```python
from build123d import *

# Parameters (mm, degrees)
EXTRUDE_1_DEPTH = 9.6
DRAFT_5_ANGLE   = -15


with BuildPart() as part:
    # 草图1 → 凸台-拉伸1 (new body)
    with BuildSketch(Plane.XY):
        Polygon((9.8, 0), (0, 0), (0, -108.97), (49.6, -108.97), (49.6, 0), (39.8, 0), (39.8, -10), (9.8, -10), align=None)
    extrude(amount=EXTRUDE_1_DEPTH)

    # 拔模5
    draft_5_faces = [part.faces().sort_by_distance(p)[0] for p in [
        (24.8, -10, 4.8),
    ]]
    draft(draft_5_faces, Plane.XY.offset(9.6), DRAFT_5_ANGLE)


solid = part.part
```
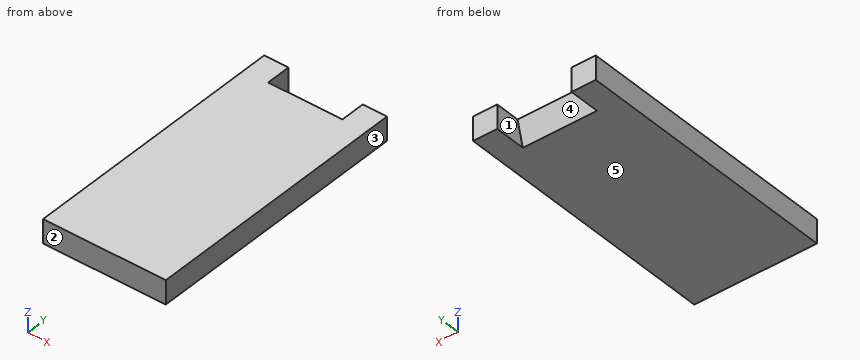
Input: part model. Units: mm. Frame: model coordinates. Face numbers are marked on the shaded views. A direction names the side the tool comes from. Coordinates: 2 decimals unless noted, no trailing zeros. Loops run counter-clockwise (first coordinate to the right, second up) from the corner with the lowest first, then second, coordinate; pieces in that order, holes last. Notation, with made-up numbers: (72.25, 72.25) - (96.25, 72.25) arc R5 cw to (96.25, 80.25) - close; hole circle Ø8 at (63.25, 8.25). An arc over 180 degrees is marked (long way). Answer in a Markdown table with one row per item.
(1) Cut plane C-C on x = 36.5. Output: boundary loops of the cut face in (y, z), plus the area to 3 significant figures.
Model answer:
| item | result |
|---|---|
| outline | (-108.97, 0) - (-12.57, 0) - (-10, 9.6) - (-108.97, 9.6) - close |
| area | 938 mm² |
(2) Cut plane D-D on z = 7.25. Output: boundary loops of the cut face in (x, y), plus the area to 3 significant figures.
Model answer:
| item | result |
|---|---|
| outline | (0, -108.97) - (49.6, -108.97) - (49.6, 0) - (39.8, 0) - (39.8, -10.63) - (9.8, -10.63) - (9.8, 0) - (0, 0) - close |
| area | 5,090 mm² |
(3) Cut plane B-B on z = 3. Output: boundary loops of the cut face in (x, y).
Model answer:
| item | result |
|---|---|
| outline | (0, -108.97) - (49.6, -108.97) - (49.6, 0) - (39.8, 0) - (39.8, -11.77) - (9.8, -11.77) - (9.8, 0) - (0, 0) - close |
(4) Cut plane A-A on y = -8. Output: boundary loops of the cut face in (x, z), plus the area to 3 significant figures.
Model answer:
| item | result |
|---|---|
| outline | (0, 0) - (9.8, 0) - (9.8, 9.6) - (0, 9.6) - close; (39.8, 0) - (49.6, 0) - (49.6, 9.6) - (39.8, 9.6) - close |
| area | 188 mm² |
(5) Set-up query: the marked faces 4 and 5. Return all of +Z, -Z, +X, -X, +Y, -Y with unobstructed straight access to the full face (end or side cutting, diameter ignored); none if empty.
Model answer:
| item | result |
|---|---|
| face 4 | -Z, +Y |
| face 5 | -Z, +X, -X, +Y, -Y |
(6) Mould query, pull axis X, two halves, no side actions, for the marked faces 1, 2 and 3. Classes: pulls with the +X half, pulls with the -X half, needs draft (parallel to the pull), parting line crosses it, or undercut.
Model answer:
| item | result |
|---|---|
| face 1 | undercut |
| face 2 | needs draft |
| face 3 | pulls with the +X half |
(7) Material intervals for L1, parallel to X at y = -8, z = 7; L2, parallel to Y at x = 37.5, z = 3.5; L3, parallel to Y at x = 11.5, z = 2, sorted ascending. Write a range as from..to.
Model answer:
| item | result |
|---|---|
| L1 | x = 0..9.8, 39.8..49.6 |
| L2 | y = -108.97..-11.63 |
| L3 | y = -108.97..-12.04 |
